Autodesk Inventor part; units mm, degrees
ref_plane "Work Plane4" through (91.948, 37.861, 63.9327) normal (0, 0.258819, 0.9659258) x (-1, 0, 0)
ref_plane "YZ Plane" through (0, 0, 0) normal (1, 0, 0) x (0, 1, 0)
ref_plane "XZ Plane" through (0, 0, 0) normal (0, 1, 0) x (-1, 0, 0)
sketch "Sketch1" plane through (0, 0, 0) normal (0, 0, 1) x (1, 0, 0)
  line L0 (0, 41.148) -> (91.948, 41.148)
  line L1 (91.948, -3.048) -> (0, -3.048)
  line L2 (0, 38.1) -> (0, 41.148)
  line L3 (0, 0) -> (0, -3.048)
  line L4 (88.9, 38.1) -> (91.948, 38.1)
  line L5 (88.9, 0) -> (91.948, 0)
  line L6 (91.948, 38.1) -> (91.948, 41.148)
  line L7 (91.948, 0) -> (91.948, -3.048)
  line L8 (45.974, 38.1) -> (45.974, 0)
  line L9 (49.022, 38.1) -> (49.022, 0)
  line L10 (88.9, 38.1) -> (49.022, 38.1)
  line L11 (45.974, 38.1) -> (0, 38.1)
  line L12 (0, 0) -> (45.974, 0)
  line L13 (49.022, 0) -> (88.9, 0)
  dimension "d0" = 88.9
  dimension "d17" = 3.048
extrude "Extrusion6" add sketch "Sketch1" along normal blind 76.2
ref_plane "Work Plane4" through (91.948, 37.861, 63.9327) normal (0, 0.258819, 0.9659258) x (-1, 0, 0)
ref_plane "Work Plane3" through (91.948, 41.148, 76.2) normal (0, 0.258819, 0.9659258) x (-1, 0, 0)
sketch "Sketch6" plane through (91.948, 37.861, 63.9327) normal (0, 0.258819, 0.9659258) x (-1, 0, 0)
  line L0 (-2.4638, -7.3313) -> (94.6916, -7.3313)
  line L1 (94.6916, -7.3313) -> (94.6916, 43.8286)
  line L2 (94.6916, 43.8286) -> (-2.4638, 43.8286)
  line L3 (-2.4638, 43.8286) -> (-2.4638, -7.3313)
  point P0 (91.948, 20.0239)
extrude "Extrusion7" cut sketch "Sketch6" along normal blind 25.4
sketch "Sketch7" plane through (45.974, 0, 0) normal (-1, 0, 0) x (0, 0, 1)
  line L0 (0, 38.1) -> (63.8687, 38.1)
  line L1 (62.4717, 38.1) -> (63.7417, 38.1)
  line L2 (63.7417, 38.1) -> (63.7417, 36.83)
  line L3 (63.7417, 36.83) -> (62.4717, 36.83)
  line L4 (62.4717, 36.83) -> (62.4717, 38.1)
  dimension "d24" = 1.27
  dimension "d25" = 1.27
  dimension "d26" = 0.127
extrude "Extrusion8" add sketch "Sketch7" along normal blind 1.27 and the other way blind 4.318
sketch "Sketch8" plane through (91.948, 37.861, 63.9327) normal (0, 0.258819, 0.9659258) x (1, 0, 0)
  line L0 (-91.948, 3.403) -> (0, 3.403)
  line L1 (-45.974, 3.403) -> (-42.926, 3.403)
  line L2 (-42.926, 3.403) -> (-42.926, 5.2369)
  line L3 (-42.926, 5.2369) -> (-45.974, 5.2369)
  line L4 (-45.974, 5.2369) -> (-45.974, 3.403)
  point P0 (-91.948, -20.0239)
extrude "Extrusion9" add sketch "Sketch8" against normal blind 12.7
sketch "Sketch10" plane through (45.974, 0, 0) normal (-1, 0, 0) x (0, 0, 1)
  line L0 (58.1292, 9.2578) -> (60.6692, 9.2578)
  line L1 (60.6692, 9.2578) -> (60.6692, 28.3078)
  line L2 (60.6692, 28.3078) -> (58.1292, 28.3078)
  line L3 (58.1292, 28.3078) -> (58.1292, 9.2578)
  dimension "d40" = 2.54
  dimension "d41" = 19.05
extrude "Extrusion11" add sketch "Sketch10" along normal blind 12.7 and the other way blind 16.51 draft 0.62
properties part number "2p1rim1" material "Steel, Galvanized"
Work out the finished part from the listing and answer in its coordinate system (mm). A direction names the side the tool comes from. Give positions to 0.01 mm unless a question says otherwise; leave off trailing zeros. Loops run counter-clockwise (first coordinate to the right, second up) from the corner with the lowest first, then second, coordinate; pieces in that order, holes last. Notation, with made-up numbers: (75.25, 48.5) -> (83.25, 48.5) arc R23 ccw to (83.25, 70.5) -> close; hole circle Ø4 at (66, -10.75). An arc over 180 degrees is marked (long way). One line per question, with ' | ' between items. Start each with the question number.
1) Section A-A, the plane x = 34.5 is taken. Determine the outline of the cut face in (y, z).
2) Section D-D, the plane y = 21 is taken. Determine the outline of the cut face in (x, z).
3) Straight lines are drawn through the part: L1, parallel to Y at x = 40.5, z = 49.5; L2, parallel to X at y = 36, z = 42; L3, parallel to X at y = 19.5, z = 60. For each, find the intervals that lie inside material, in ascending order.
4) Each of these flat-tipped pins is pushed along its axis until it touches: pin 1 (0.6 mm diameter, centred on x = 49.5, y = 37.5, fed in from +Z); pin 2 (0.5 mm diameter, centred on y = 42, z = 60.5, fed in from -X); pin 3 (1 mm diameter, centred on x = 28, y = 36.5, fed in from +Z); pin 4 (5 mm diameter, centred on x = 63.5, z = 18, fed in from +Y). Where does it stop, or does it pass through?
5) Section C-C, the plane z = 44.5 is taken. Determine the outline of the cut face in (x, y), then the cut area to 3 significant figures.
6) For faces 1 (the face through (40, 19, 60.669)), 2 (the face through (70, 0, 37)), 3 (the face through (33.274, 19, 59)), 4 (the face through (40, 19, 58.129)), determine the directions among +Z, -Z, +X, -X, +Y, -Y from which every point of the face is accessible in a straight line to the end or side of a thin tool.
7) Section B-B, the plane x = 67.5 is taken. Determine the outline of the cut face in (y, z), then the cut area to 3 significant figures.
Resolved:
1) outline: (-3.05, 0) -> (0, 0) -> (0, 74.08) -> (-3.05, 74.89) -> close; (9.26, 58.13) -> (28.31, 58.13) -> (28.31, 60.67) -> (9.26, 60.67) -> close; (38.1, 0) -> (41.15, 0) -> (41.15, 63.05) -> (38.1, 63.87) -> close
2) outline: (33.27, 58.13) -> (45.97, 58.13) -> (45.97, 0) -> (49.02, 0) -> (49.02, 58.1) -> (62.48, 57.95) -> (62.48, 60.85) -> (49.02, 60.7) -> (49.02, 68.45) -> (45.97, 68.45) -> (45.97, 60.67) -> (33.27, 60.67) -> close
3) L1: -3.05 to 0, 38.1 to 41.15 | L2: 45.97 to 49.02 | L3: 33.27 to 62.48
4) pin 1: z = 63.74 | pin 2: x = 45.97 | pin 3: through | pin 4: y = 41.15
5) outline: (0, -3.05) -> (91.95, -3.05) -> (91.95, 0) -> (49.02, 0) -> (49.02, 38.1) -> (91.95, 38.1) -> (91.95, 41.15) -> (0, 41.15) -> (0, 38.1) -> (45.97, 38.1) -> (45.97, 0) -> (0, 0) -> close | area: 677 mm2
6) face 1: +Z, -X | face 2: +Z, -Z, +X | face 3: +Z, -Z, -X | face 4: -Z, -X
7) outline: (-3.05, 0) -> (0, 0) -> (0, 74.08) -> (-3.05, 74.89) -> close; (38.1, 0) -> (41.15, 0) -> (41.15, 63.05) -> (38.1, 63.87) -> close | area: 420 mm2
